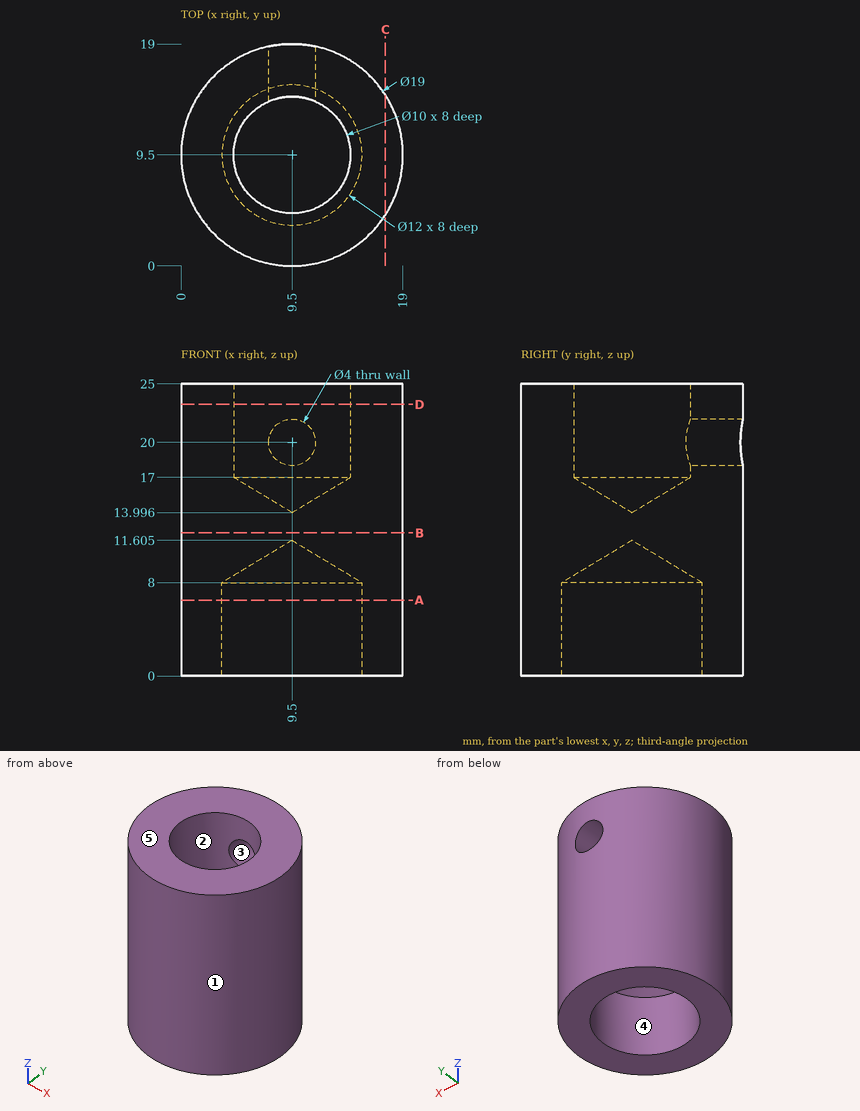
The figure shows three views and two pictorial views of one solid part (mm, origin at its lowest corner). Answer the questions. A direction names the side the tool comes from. Round coordinates to 2 decimals unless told otherwise and drop trailing zeros. Loops run counter-clockwise (first coordinate to the right, second up) from the corner with the lowest first, then second, coordinate; pieces in that order, holes last. Notation, with made-up numbers: M 80.5,-33 L 102.5,-33 A26 cw 102.5,-13 Z; hole C 51,-34 d5. An arc over 180 degrees is marked long. Return JSON: item names as keys, results as strings.
Q1. The mould has two halves that part along Z. Classify the marked faces 3, 4 and 5: released by +Z, released by -Z, zero draft, split by the parting line, or undercut.
Results list:
{"face 3": "undercut", "face 4": "zero draft", "face 5": "released by +Z"}
Q2. Each of these flat-tipped pins is pushed along its axis until it touches: pin 1 Ø2 at (x, y) = (11.5, 10.5) entering from +Z; pin 2 Ø2 at (x, y) = (7, 7.5) entering from -Z; pin 3 Ø10 at (x, z) = (3.5, 8) entering from -Y. Where does it stop, or does it pass through?
Results list:
{"pin 1": "stops at z = 15.94", "pin 2": "stops at z = 9.08", "pin 3": "stops at y = 0.05"}
Q3. Find section C-C, the plane x = 17.5. Determine the outline of the cut face in (y, z), plus the area to 3 significant figures.
Results list:
{"outline": "M 4.38,0 L 14.62,0 L 14.62,25 L 4.38,25 Z", "area": "256 mm2"}
Q4. Find the intervals of material crossed by line 1 along Y through (x, z) = (9.75, 3.5) (1 decimal); line 2 along Z through (x, y) = (9.5, 16); line 3 along X through (y, z) = (11, 2.25), in increasing order. Write a range as from..to.
Results list:
{"line 1": "y = 0..3.5, 15.5..19", "line 2": "z = 0..18, 22..25", "line 3": "x = 0.12..3.69, 15.31..18.88"}
Q5. Which of the six approach directions +Z, -Z, +X, -X, +Y, -Y give full straight-line access (tool end or side, diameter ignored) to the marked faces 1 and 2?
Results list:
{"face 1": "+Z, -Z", "face 2": "+Z"}
Q6. Find section D-D, the plane z = 23.25. Determine the outline of the cut face in (x, y).
Results list:
{"outline": "C 9.5,9.5 d19; hole C 9.5,9.5 d10"}
Q7. Find section B-B, the plane z = 12.25. Determine the outline of the cut face in (x, y).
Results list:
{"outline": "C 9.5,9.5 d19"}
Q8. Find section A-A, the plane z = 6.5. Determine the outline of the cut face in (x, y), plus the area to 3 significant figures.
Results list:
{"outline": "C 9.5,9.5 d19; hole C 9.5,9.5 d12", "area": "170 mm2"}
